Part model, mm, in its own coordinate system. A direction names the side the tool comes from. Coordinates: 2 decimals unless noted, no trailing zeros. Loops run counter-clockwise (first coordinate to the right, second up) from the corner with the lowest first, then second, coordinate; pieces in that order, holes last. Notation, with made-up numbers: (46, 71) -> (54, 71) arc R20 ccw to (54, 80) -> close; hole circle Ø7 at (-24, 24). An arc over 180 degrees is marked (long way). Use one line per item in the form item = value. Start each with the question number.
(1) 3-axis set-ups, long thin cutter, end or side, ignore diameter. For faces 1 (the cylindrical face through (-24.75, 0.81, -87.77)), 2 (the flat face through (-1, 1.6, -18)), 3 (the cylindrical face through (-18.77, 0.79, 48.89)): which of +Z, -Z, +X, -X, +Y, -Y reach the whole face in a straight line?
(2) Band-saw the part on B-B on x = -2. Give the cut face in (y, z), then the cut area to 3 significant figures.
(3) Band-saw the part on C-C on y = 0.8. Count the separate pieces of the cut face and the enclosed holes in it, then the cut area to 3 significant figures.
(4) Drill centre lines: L1, parallel to X at y = 0.7, z = -42; L2, parallel to X at y = 0.9, z = -79; L3, parallel to Z at x = 5.5, y = 1.55. Where is each one in solid material? Low to high. Write a range as [from, to].
(5) Mould opens along X. For faces 4 (the flat face through (39, 0.8, -84.4)), 5 (the cylindrical face through (23.2, 0.789, 19.715)), 6 (the flat face through (-38.91, 0.79, -84.55)) say: +X half, -X half, draft (parallel to the pull), parting line (faces both ways), or undercut.
(6) Band-saw the part on A-A on z = -44.5. Give the cut face in (x, y).
(7) Pin check, flat tip, straight feed: P1, Ø0.5, axis at x = 10, y = 1, coming from the -Z side. Stop position of the tip, or through.
```python
from build123d import *

# Parameters (mm, degrees)
SKETCH1_W               = 2.1
SKETCH1_H               = 8.5
SKETCH1_R               = 1.55
EXTRUDE_8657_DEPTH      = 1.6
CUT_EXTRUDE_9042_DEPTH  = 98.639296877
CUT_EXTRUDE_9381_DEPTH  = 98.639296877
CUT_EXTRUDE_9654_DEPTH  = 10
FILLET_1_R              = 2.5
SKETCH_9947_R           = 0.5
CUT_EXTRUDE_10465_DEPTH = 98.639296877


with BuildPart() as part:
    # Sketch1 → Extrude 8657 (new body)
    with BuildSketch(Plane(origin=(0, 0, 0), x_dir=(1, 0, 0), z_dir=(0, 1, 0))):
        with BuildLine():
            Line((-41.25, 0), (-41.25, -55))
            Line((-41.25, -55), (-34.369560329, -55))
            ThreePointArc((-34.369560329, -55), (-18.59120626, -48.721265785), (-11.440696816, -33.31837076))
            ThreePointArc((-11.440696816, -33.31837076), (-7.872843983, -25.632867641), (0, -22.5))
            ThreePointArc((0, -22.5), (7.872843983, -25.632867641), (11.440696816, -33.31837076))
            ThreePointArc((11.440696816, -33.31837076), (18.59120626, -48.721265785), (34.369560329, -55))
            Line((34.369560329, -55), (41.25, -55))
            Line((41.25, -55), (41.25, 0))
            Line((41.25, 0), (41.25, 80.5))
            Line((41.25, 80.5), (36.640789302, 88.483387111))
            Line((36.640789302, 88.483387111), (-36.640789302, 88.483387111))
            Line((-36.640789302, 88.483387111), (-41.25, 80.5))
            Line((-41.25, 80.5), (-41.25, 0))
        make_face()
        with Locations((-36.8, -46.75)):
            Rectangle(SKETCH1_W, SKETCH1_H, mode=Mode.SUBTRACT)
        with Locations(Location((-32.325, -35, 0), (0, 0, 270))):
            Circle(SKETCH1_R, mode=Mode.SUBTRACT)
        with Locations(Location((-17.5, -36.97765453, 0), (0, 0, 270))):
            Circle(SKETCH1_R, mode=Mode.SUBTRACT)
        with Locations((-36.8, -16.75)):
            Rectangle(SKETCH1_W, SKETCH1_H, mode=Mode.SUBTRACT)
        with Locations(Location((-24.575, -19, 0), (0, 0, 270))):
            Circle(SKETCH1_R, mode=Mode.SUBTRACT)
        with Locations(Location((17.5, -36.97765453, 0), (0, 0, 270))):
            Circle(SKETCH1_R, mode=Mode.SUBTRACT)
        with Locations((36.8, -46.75)):
            Rectangle(SKETCH1_W, SKETCH1_H, mode=Mode.SUBTRACT)
        with Locations(Location((32.325, -35, 0), (0, 0, 270))):
            Circle(SKETCH1_R, mode=Mode.SUBTRACT)
        with Locations(Location((24.575, -19, 0), (0, 0, 270))):
            Circle(SKETCH1_R, mode=Mode.SUBTRACT)
        with Locations((36.8, -16.75)):
            Rectangle(SKETCH1_W, SKETCH1_H, mode=Mode.SUBTRACT)
        with Locations((-36.8, 43.25)):
            Rectangle(SKETCH1_W, SKETCH1_H, mode=Mode.SUBTRACT)
        with Locations(Location((-32.325, 52.5, 0), (0, 0, 270))):
            Circle(SKETCH1_R, mode=Mode.SUBTRACT)
        with Locations(Location((-24.575, 39, 0), (0, 0, 270))):
            Circle(SKETCH1_R, mode=Mode.SUBTRACT)
        with Locations((-36.8, 73.25)):
            Rectangle(SKETCH1_W, SKETCH1_H, mode=Mode.SUBTRACT)
        with Locations(Location((-15.000000144, 64.02234547, 0), (0, 0, 270))):
            Circle(SKETCH1_R, mode=Mode.SUBTRACT)
        with Locations(Location((24.575, 39, 0), (0, 0, 270))):
            Circle(SKETCH1_R, mode=Mode.SUBTRACT)
        with Locations((36.8, 43.25)):
            Rectangle(SKETCH1_W, SKETCH1_H, mode=Mode.SUBTRACT)
        with Locations(Location((32.325, 52.5, 0), (0, 0, 270))):
            Circle(SKETCH1_R, mode=Mode.SUBTRACT)
        Polygon((7.65, 60.772345), (7.65, 82.35), (23.6, 82.35), (23.6, 55.25), (15.4, 55.25), (15.4, 60.772345), align=None, mode=Mode.SUBTRACT)
        with Locations((36.8, 73.25)):
            Rectangle(SKETCH1_W, SKETCH1_H, mode=Mode.SUBTRACT)
    extrude(amount=EXTRUDE_8657_DEPTH)

    # 外部切除点示意-1 → Cut-Extrude 9042 (cut, through all)
    with BuildSketch(Plane(origin=(0, 0, 0), x_dir=(1, 0, 0), z_dir=(0, 1, 0))):
        with BuildLine():
            Line((-41.25, 28.319513771), (-41.285942601, -7.350545872))
            ThreePointArc((-41.285942601, -7.350545872), (-37.250021115, 10.480435299), (-41.25, 28.319513771))
        make_face()
        with BuildLine():
            Line((41.25, 28.319513771), (41.285942601, -7.350545872))
            ThreePointArc((41.285942601, -7.350545872), (37.250021115, 10.480435299), (41.25, 28.319513771))
        make_face()
        Polygon((5.1, 67.733387111), (7.65, 67.733387111), (7.65, 82.35), (23.6, 82.35), (23.6, 88.483387111), (5.1, 88.483387111), (-24, 88.483387111), (-24, 67.733387111), align=None)
    extrude(amount=CUT_EXTRUDE_9042_DEPTH, mode=Mode.SUBTRACT)

    # Sketch 9088 → Cut-Extrude 9381 (cut, through all)
    with BuildSketch(Plane(origin=(0, 0, 0), x_dir=(1, 0, 0), z_dir=(0, 1, 0))):
        with BuildLine():
            Line((-30.25, 20.025), (-27.75, 20.025))
            ThreePointArc((-27.75, 20.025), (-26.475, 18.75), (-27.75, 17.475))
            Line((-27.75, 17.475), (-30.25, 17.475))
            ThreePointArc((-30.25, 17.475), (-31.525, 18.75), (-30.25, 20.025))
        make_face()
        with BuildLine():
            Line((-6.75, 20.025), (-9.25, 20.025))
            ThreePointArc((-9.25, 20.025), (-10.525, 18.75), (-9.25, 17.475))
            Line((-9.25, 17.475), (-6.75, 17.475))
            ThreePointArc((-6.75, 17.475), (-5.475, 18.75), (-6.75, 20.025))
        make_face()
        with BuildLine():
            Line((-30.25, -2.525), (-27.75, -2.525))
            ThreePointArc((-27.75, -2.525), (-26.475, -1.25), (-27.75, 0.025))
            Line((-27.75, 0.025), (-30.25, 0.025))
            ThreePointArc((-30.25, 0.025), (-31.525, -1.25), (-30.25, -2.525))
        make_face()
        with BuildLine():
            Line((-6.75, -2.525), (-9.25, -2.525))
            ThreePointArc((-9.25, -2.525), (-10.525, -1.25), (-9.25, 0.025))
            Line((-9.25, 0.025), (-6.75, 0.025))
            ThreePointArc((-6.75, 0.025), (-5.475, -1.25), (-6.75, -2.525))
        make_face()
    extrude(amount=CUT_EXTRUDE_9381_DEPTH, mode=Mode.SUBTRACT)

    # 草图2 → Cut-Extrude 9654 (cut)
    with BuildSketch(Plane(origin=(0, 1.6, 0), x_dir=(1, 0, 0), z_dir=(0, 1, 0))):
        with BuildLine():
            ThreePointArc((9.371867176, 10.52234547), (19.323145451, 20.402758988), (29.820182402, 29.701292521))
            ThreePointArc((29.820182402, 29.701292521), (26.696086154, 10.52234547), (29.820182402, -8.65660158))
            ThreePointArc((29.820182402, -8.65660158), (19.323145451, 0.641931952), (9.371867176, 10.52234547))
        make_face()
        with BuildLine():
            ThreePointArc((0, 1.150478295), (9.880413518, -8.800799981), (19.178947051, -19.297836932))
            ThreePointArc((19.178947051, -19.297836932), (0, -16.173740684), (-19.178947051, -19.297836932))
            ThreePointArc((-19.178947051, -19.297836932), (-9.880413518, -8.800799981), (0, 1.150478295))
        make_face()
        with BuildLine():
            ThreePointArc((0, 19.894212646), (-9.880413518, 29.845490922), (-19.178947051, 40.342527872))
            ThreePointArc((-19.178947051, 40.342527872), (0, 37.218431624), (19.178947051, 40.342527872))
            ThreePointArc((19.178947051, 40.342527872), (9.880413518, 29.845490922), (0, 19.894212646))
        make_face()
    extrude(amount=-CUT_EXTRUDE_9654_DEPTH, mode=Mode.SUBTRACT)

    # 圆角1
    fillet_1_edges = [part.edges().sort_by_distance(p)[0] for p in [
        (23.6, 0.8, -88.483387111),
        (-24, 0.8, -88.483387111),
        (-24, 0.8, -67.733387111),
    ]]
    fillet(fillet_1_edges, radius=FILLET_1_R)

    # Sketch 9947 → Cut-Extrude 10465 (cut, through all)
    with BuildSketch(Plane(origin=(0, 0, 0), x_dir=(1, 0, 0), z_dir=(0, 1, 0))):
        with Locations((7.65, 60.772345)):
            Circle(SKETCH_9947_R)
        with Locations((15.4, 60.772345)):
            Circle(SKETCH_9947_R)
        with Locations((15.4, 55.25)):
            Circle(SKETCH_9947_R)
        with Locations((23.6, 55.25)):
            Circle(SKETCH_9947_R)
        with Locations((35.75, 69)):
            Circle(SKETCH_9947_R)
        with Locations((37.85, 69)):
            Circle(SKETCH_9947_R)
        with Locations((35.75, 77.5)):
            Circle(SKETCH_9947_R)
        with Locations((37.85, 77.5)):
            Circle(SKETCH_9947_R)
        with Locations((35.75, 47.5)):
            Circle(SKETCH_9947_R)
        with Locations((37.85, 47.5)):
            Circle(SKETCH_9947_R)
        with Locations((35.75, 39)):
            Circle(SKETCH_9947_R)
        with Locations((37.85, 39)):
            Circle(SKETCH_9947_R)
        with Locations((35.75, -12.5)):
            Circle(SKETCH_9947_R)
        with Locations((37.85, -12.5)):
            Circle(SKETCH_9947_R)
        with Locations((35.75, -21)):
            Circle(SKETCH_9947_R)
        with Locations((37.85, -21)):
            Circle(SKETCH_9947_R)
        with Locations((35.75, -42.5)):
            Circle(SKETCH_9947_R)
        with Locations((37.85, -42.5)):
            Circle(SKETCH_9947_R)
        with Locations((35.75, -51)):
            Circle(SKETCH_9947_R)
        with Locations((37.85, -51)):
            Circle(SKETCH_9947_R)
        with Locations((-37.85, -51)):
            Circle(SKETCH_9947_R)
        with Locations((-35.75, -51)):
            Circle(SKETCH_9947_R)
        with Locations((-37.85, -42.5)):
            Circle(SKETCH_9947_R)
        with Locations((-35.75, -42.5)):
            Circle(SKETCH_9947_R)
        with Locations((-37.85, -21)):
            Circle(SKETCH_9947_R)
        with Locations((-35.75, -21)):
            Circle(SKETCH_9947_R)
        with Locations((-37.85, -12.5)):
            Circle(SKETCH_9947_R)
        with Locations((-35.75, -12.5)):
            Circle(SKETCH_9947_R)
        with Locations((-37.85, 39)):
            Circle(SKETCH_9947_R)
        with Locations((-35.75, 39)):
            Circle(SKETCH_9947_R)
        with Locations((-37.85, 47.5)):
            Circle(SKETCH_9947_R)
        with Locations((-35.75, 47.5)):
            Circle(SKETCH_9947_R)
        with Locations((-37.85, 77.5)):
            Circle(SKETCH_9947_R)
        with Locations((-35.75, 77.5)):
            Circle(SKETCH_9947_R)
        with Locations((-37.85, 69)):
            Circle(SKETCH_9947_R)
        with Locations((-35.75, 69)):
            Circle(SKETCH_9947_R)
    extrude(amount=CUT_EXTRUDE_10465_DEPTH, mode=Mode.SUBTRACT)


solid = part.part
```
A:
q1.face_1 = -Z, +Y, -Y
q1.face_2 = +Z, -Z, +X, -X, +Y
q1.face_3 = +Z, +Y, -Y
q2.outline = (0, -67.73) -> (1.6, -67.73) -> (1.6, -37.25) -> (0, -37.25) -> close; (0, -21.82) -> (1.6, -21.82) -> (1.6, 0.77) -> (0, 0.77) -> close; (0, 16.21) -> (1.6, 16.21) -> (1.6, 22.68) -> (0, 22.68) -> close
q2.area = 95.3 mm²
q3.separate_pieces = 1
q3.enclosed_holes = 26
q3.area = 8,280 mm²
q4.L1 = [-41.25, -37.85], [-35.75, 35.75], [37.85, 41.25]
q4.L2 = [-41.25, -24], [23.6, 41.25]
q4.L3 = [-67.73, -37.47], [-25.29, 4.25], [16.42, 23.91]
q5.face_4 = +X half
q5.face_5 = undercut
q5.face_6 = -X half
q6.outline = (-41.25, 0) -> (-37.85, 0) -> (-37.85, 1.6) -> (-41.25, 1.6) -> close; (-35.75, 0) -> (35.75, 0) -> (35.75, 1.6) -> (-35.75, 1.6) -> close; (37.85, 0) -> (41.25, 0) -> (41.25, 1.6) -> (37.85, 1.6) -> close
q7.P1 = -60.77
